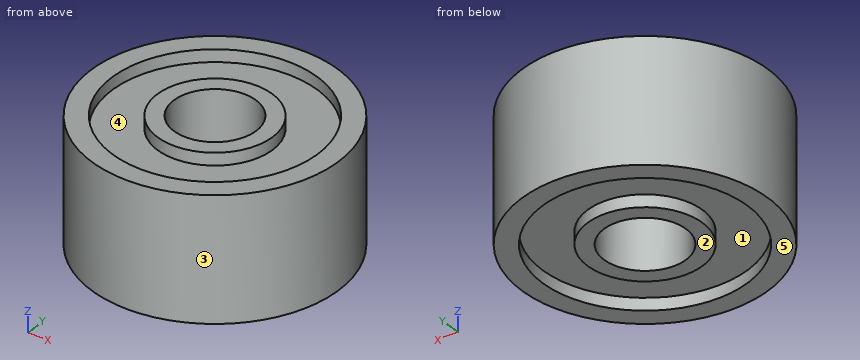
```python
from build123d import *

# Parameters (mm, degrees)
SKETCH1_R           = 3
SKETCH1_R_2         = 1
BOSS_EXTRUDE1_DEPTH = 3
SKETCH2_R           = 2.5
SKETCH2_R_2         = 1.4
CUT_EXTRUDE1_DEPTH  = 0.3
CUT_EXTRUDE2_START  = -3
SKETCH2_2_R         = 2.5
SKETCH2_2_R_2       = 1.4
CUT_EXTRUDE2_DEPTH  = 0.3


with BuildPart() as part:
    # Sketch1 → Boss-Extrude1 (new body)
    with BuildSketch(Plane.XY):
        Circle(SKETCH1_R)
        Circle(SKETCH1_R_2, mode=Mode.SUBTRACT)
    extrude(amount=BOSS_EXTRUDE1_DEPTH)

    # Sketch2 → Cut-Extrude1 (cut)
    with BuildSketch(Plane.XY.offset(3)):
        Circle(SKETCH2_R)
        Circle(SKETCH2_R_2, mode=Mode.SUBTRACT)
    extrude(amount=-CUT_EXTRUDE1_DEPTH, mode=Mode.SUBTRACT)

    # Sketch2<2> → Cut-Extrude2 (cut)
    with BuildSketch(Plane.XY.offset(3).offset(CUT_EXTRUDE2_START)):
        Circle(SKETCH2_2_R)
        Circle(SKETCH2_2_R_2, mode=Mode.SUBTRACT)
    extrude(amount=CUT_EXTRUDE2_DEPTH, mode=Mode.SUBTRACT)


solid = part.part
```
Geometry check sheet. Reference: the model listing, model coordinates, mm. Face numbers are marked on the shaded views. A direction names the side the tool comes from. Coordinates: 2 decimals unless noted, no trailing zeros. Loops run counter-clockwise (first coordinate to the right, second up) from the corner with the lowest first, then second, coordinate; pieces in that order, holes last.
Item 1: Thickness scan on line 1 (Y direction, x = 0, z = 2.95); line 2 (Y direction, x = 0, z = 1.35); line 3 (Z direction, x = 2.1, y = -0.3). Record the ranges inside material, lowest first.
Item 2: Sectioned sample at C-C, the plane z = 2.05. Record the boundary of the cut face in (x, y).
Item 3: Go/stop test with a flat-tipped pin: pin 1 Ø1 at (y, z) = (-2.5, 1) entering from +X. Record where the tip stops, or that it passes through.
Item 4: Sectioned sample at D-D, the plane x = -1.7. Record the boundary of the cut face in (y, z), then the cut area to 3 significant figures.
Item 5: Access from +Z, -Z, +X, -X, +Y, -Y to the whole of each face (thin tool, end or side, straight path). Record for the marked faces 1 and 2.
Item 6: Release check for a two-part mould opening along Y. For the marked faces 3, 4 and 5 record: released by +Y, released by -Y, zero draft, split by the parting line, or undercut.
Item 7: Sectioned sample at A-A, the plane x = 0. Record the boundary of the cut face in (y, z).
Check result:
1. line 1: y = -3 to -2.5, -1.4 to -1, 1 to 1.4, 2.5 to 3
1. line 2: y = -3 to -1, 1 to 3
1. line 3: z = 0.3 to 2.7
2. outline: circle Ø6 at (0, 0); hole circle Ø2 at (0, 0)
3. pin 1: stops at x = 2.24
4. outline: (-2.47, 0) - (-1.83, 0) - (-1.83, 0.3) - (1.83, 0.3) - (1.83, 0) - (2.47, 0) - (2.47, 3) - (1.83, 3) - (1.83, 2.7) - (-1.83, 2.7) - (-1.83, 3) - (-2.47, 3) - close
4. area: 12.6 mm2
5. face 1: -Z
5. face 2: -Z, +X, -X, +Y, -Y
6. face 3: split by the parting line
6. face 4: undercut
6. face 5: zero draft
7. outline: (-3, 0) - (-2.5, 0) - (-2.5, 0.3) - (-1.4, 0.3) - (-1.4, 0) - (-1, 0) - (-1, 3) - (-1.4, 3) - (-1.4, 2.7) - (-2.5, 2.7) - (-2.5, 3) - (-3, 3) - close; (1, 0) - (1.4, 0) - (1.4, 0.3) - (2.5, 0.3) - (2.5, 0) - (3, 0) - (3, 3) - (2.5, 3) - (2.5, 2.7) - (1.4, 2.7) - (1.4, 3) - (1, 3) - close
